Source: CAD feature listing. Evaluate the final solid. Frame: model axes, mm. Give positions to 0.01 mm unless a question says otherwise; leave off trailing zeros. Write each loop counter-clockwise with the first axis right and the second up, starting at its lowest first coordinate (ties: lowest second). Pieces come first, ordered by that corner, then holes. Notation, with made-up numbers: (15.25, 18) -> (29.25, 18) arc R25 ccw to (29.25, 53) -> close; hole circle Ø3 at (76, 13.25). An arc over 180 degrees is marked (long way). Use one line per item in the form item = value. Start each with the question number.
(1) Draft query along Y for faces 1 (the face through (-28.5, -35, 0)), 2 (the face through (0, 38.1, 0)), 3 (the face through (-14.328, 13.247, 0.022)). Return one class per face: pulls with the +Y half, pulls with the -Y half, needs draft (parallel to the pull), parting line crosses it, or undercut.
(2) Material intervals for line 1 along Y through (x, z) = (-19.05, -0.6) (3 decimals); line 2 along Y through (x, z) = (15.5, 0.8); line 3 along Y through (x, z) = (-17, -0.75), sorted ascending. Write a range as from..to.
(3) Cut plane C-C, the plane x = -19.05. Output: boundary loops of the cut face in (y, z) (1 decimal), and give its area (3 significant figures).
(4) Cut plane A-A, the plane y = 0. Output: boundary loops of the cut face in (x, z), and give its area (3 significant figures).
(5) Cut plane B-B, the plane z = 0.3. Count the separate pieces of the cut face and the enclosed holes in it, and give its area (3 significant figures).
(6) Cut plane D-D, the plane x = 0. Output: boundary loops of the cut face in (y, z).
from build123d import *

# Parameters (mm, degrees)
SKETCH1_W           = 63.5
SKETCH1_H           = 76.2
BOSS_EXTRUDE1_DEPTH = 1.5875
SKETCH2_R           = 3.175
CUT_EXTRUDE1_DEPTH  = 4.175
SKETCH3_R           = 2.54
CUT_EXTRUDE2_DEPTH  = 4.175
CHAMFER1_SIZE       = 6.35
SKETCH4_R           = 11.5
CUT_EXTRUDE3_DEPTH  = 4.175


with BuildPart() as part:
    # Sketch1 → Boss-Extrude1 (new body, symmetric)
    with BuildSketch(Plane.XY):
        Rectangle(SKETCH1_W, SKETCH1_H)
    extrude(amount=BOSS_EXTRUDE1_DEPTH, both=True)

    # Sketch2 → Cut-Extrude1 (cut, through all)
    with BuildSketch(Plane.XY.offset(1.5875)):
        with Locations((-19.05, 31.75)):
            Circle(SKETCH2_R)
        with Locations((19.05, 31.75)):
            Circle(SKETCH2_R)
        with Locations((19.05, -31.75)):
            Circle(SKETCH2_R)
        with Locations((-19.05, -31.75)):
            Circle(SKETCH2_R)
    extrude(amount=-CUT_EXTRUDE1_DEPTH, mode=Mode.SUBTRACT)

    # Sketch3 → Cut-Extrude2 (cut, through all)
    with BuildSketch(Plane.XY.offset(1.5875)):
        with Locations((-15.5, 15.5)):
            Circle(SKETCH3_R)
        with Locations((15.5, 15.5)):
            Circle(SKETCH3_R)
        with Locations((15.5, -15.5)):
            Circle(SKETCH3_R)
        with Locations((-15.5, -15.5)):
            Circle(SKETCH3_R)
    extrude(amount=-CUT_EXTRUDE2_DEPTH, mode=Mode.SUBTRACT)

    # Chamfer1
    chamfer1_edges = [part.edges().sort_by_distance(p)[0] for p in [
        (31.75, -38.1, 0),
        (-31.75, -38.1, 0),
        (-31.75, 38.1, 0),
        (31.75, 38.1, 0),
    ]]
    chamfer(chamfer1_edges, length=CHAMFER1_SIZE)

    # Sketch4 → Cut-Extrude3 (cut, through all)
    with BuildSketch(Plane.XY.offset(1.5875)):
        Circle(SKETCH4_R)
    extrude(amount=-CUT_EXTRUDE3_DEPTH, mode=Mode.SUBTRACT)


solid = part.part
Geometry says:
q1.face_1 = pulls with the -Y half
q1.face_2 = pulls with the +Y half
q1.face_3 = undercut
q2.line_1 = -38.1..-34.925, -28.575..28.575, 34.925..38.1
q2.line_2 = -38.1..-18.04, -12.96..12.96, 18.04..38.1
q2.line_3 = -38.1..-34.17, -29.33..-17.55, -13.45..13.45, 17.55..29.33, 34.17..38.1
q3.outline = (-38.1, -1.6) -> (-34.9, -1.6) -> (-34.9, 1.6) -> (-38.1, 1.6) -> close; (-28.6, -1.6) -> (28.6, -1.6) -> (28.6, 1.6) -> (-28.6, 1.6) -> close; (34.9, -1.6) -> (38.1, -1.6) -> (38.1, 1.6) -> (34.9, 1.6) -> close
q3.area = 202 mm^2
q4.outline = (-31.75, -1.59) -> (-11.5, -1.59) -> (-11.5, 1.59) -> (-31.75, 1.59) -> close; (11.5, -1.59) -> (31.75, -1.59) -> (31.75, 1.59) -> (11.5, 1.59) -> close
q4.area = 129 mm^2
q5.separate_pieces = 1
q5.enclosed_holes = 9
q5.area = 4,130 mm^2
q6.outline = (-38.1, -1.59) -> (-11.5, -1.59) -> (-11.5, 1.59) -> (-38.1, 1.59) -> close; (11.5, -1.59) -> (38.1, -1.59) -> (38.1, 1.59) -> (11.5, 1.59) -> close
